from build123d import *

# Parameters (mm, degrees)
F2_R     = 0.3
F3_DEPTH = 1.27


# Not quite as in the source:
# - a feature names something its author has since deleted; it is built from what else it names


with BuildPart() as f1:
    # F0 (on Front) → F1 (revolve)
    with BuildSketch(Plane.XZ):
        with BuildLine():
            Line((-1.87, 0), (0, 0))
            Line((0, 0), (0, 5.49))
            Line((0, 5.49), (-0.23, 5.49))
            ThreePointArc((-0.23, 5.49), (-1.1280256121, 5.1180256121), (-1.5, 4.22))
            Line((-1.5, 4.22), (-1.5, 1))
            Line((-1.5, 1), (-1.87, 1))
            Line((-1.87, 1), (-1.87, 0))
        make_face()
    revolve(axis=Axis((0, 0, 2.745), (0, 0, -1)))

    # F2 (on face) → F3 (join)
    with BuildSketch(Plane(origin=(0, 0, 0), x_dir=(1, 0, 0), z_dir=(0, 0, -1))):
        with Locations((-0.8715403965, 0)):
            Circle(F2_R)
        with Locations((0.8715403965, 0)):
            Circle(F2_R)
    extrude(amount=F3_DEPTH)


solid = f1.part
Model file for the job. Use its own axes, mm. Give positions to 0.01 mm unless a question says otherwise; leave off trailing zeros. Loops run counter-clockwise (first coordinate to the right, second up) from the corner with the lowest first, then second, coordinate; pieces in that order, holes last.
1) Saw through at B-B (z = 2). Write the cut outline in (x, y).
2) Saw through at C-C (y = 1.6). Write the cut outline in (x, z), plus the area to 3 significant figures.
3) Flat gauge pins, fed straight in: pin 1 Ø1.5 at (y, z) = (-1, 3.5) entering from +X; pin 2 Ø1.9 at (x, y) = (0, 0) entering from -Z. Where does each tip first touch, or does it go through?
4) Pull direction Z, two halves, no side cores. Call faces 1 (the cylindrical face through (0.243, 1.854, 0.493)), 2 (the flat face through (0, 0, 0)): +Z half, -Z half, draft (parallel to the pull), parting line (faces both ways), or undercut.
5) Saw through at A-A (z = -0.5). Write the cut outline in (x, y), plus the area to 3 significant figures.
6) Saw through at D-D (z = 0.25). Write the cut outline in (x, y).
7) Wall check: line 1 (Z direction, x = 1.15, y = -1.3); line 2 (Y direction, x = 0.95, z = 3.25); line 3 (X direction, y = -0.55, z = 3.5). Give the ranges that are in metal, low to high.
Answer block:
1. outline: circle Ø3 at (0, 0)
2. outline: (-0.97, 0) - (0.97, 0) - (0.97, 1) - (-0.97, 1) - close
2. area: 1.94 mm2
3. pin 1: stops at x = 1.48
3. pin 2: stops at z = -1.27
4. face 1: draft
4. face 2: -Z half
5. outline: circle Ø0.6 at (-0.87, 0); circle Ø0.6 at (0.87, 0)
5. area: 0.565 mm2
6. outline: circle Ø3.74 at (0, 0)
7. line 1: z = 0 to 1
7. line 2: y = -1.16 to 1.16
7. line 3: x = -1.4 to 1.4
